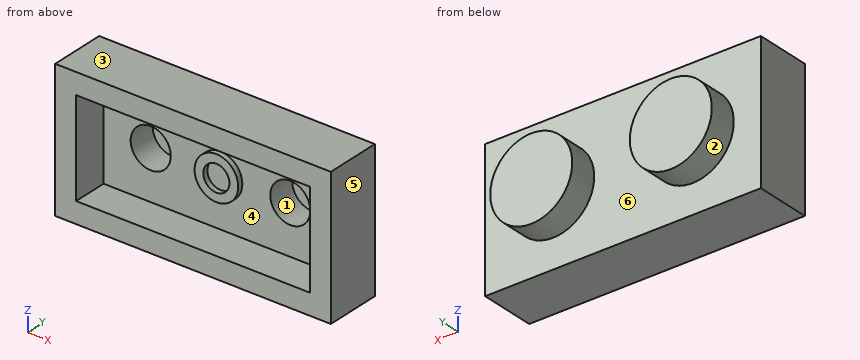
```python
from build123d import *

# Parameters (mm, degrees)
MAINBASESKETCH_W        = 15.8
MAINBASESKETCH_H        = 3.2
MAINBASEEXTRUDE_DEPTH   = 7.9
STUDSSKETCH_R           = 2.35
STUDSEXTRUDE_DEPTH      = 1.6
STUDSPATTERN_COUNT      = 2
STUDSPATTERN_PITCH      = 8
STUDSPATTERN_COUNT_DIR2 = 2
STUDSPATTERN_PITCH_DIR2 = 8
MAINBASESHELL_T         = -1.2
LCUTBLUE_DEPTH          = 19.555463972
LCUTBLUE_DEPTH_BACK     = 19.555463972
CUTADDEDTOLCUT_DEPTH    = 2
MADESLIMCUTSKETCH_W     = 7.9
MADESLIMCUTSKETCH_H     = 7.9
MADESLIMCUT_DEPTH       = 19.897228453
MADESLIMFILLEXT_REACH   = 20.897
SKETCH33_W              = 5.500952983
SKETCH33_H              = 1.199047018
SLIMHOLEEXT_START       = -0.2
SLIMHOLESKETCH_R        = 1.25
SLIMHOLESKETCH_R_2      = 0.75
SLIMHOLEEXT_DEPTH       = 0.5


with BuildPart() as part:
    # MainBaseSketch → MainBaseExtrude (new, symmetric)
    with BuildSketch(Plane.XY):
        with Locations((8.581967213, 1.6)):
            Rectangle(MAINBASESKETCH_W, MAINBASESKETCH_H)
    extrude(amount=MAINBASEEXTRUDE_DEPTH, both=True)

    # StudsSketch → StudsExtrude (add)
    with BuildSketch(Plane(origin=(0, 3.2, 0), x_dir=(1, 0, 0), z_dir=(0, 1, 0))):
        with Locations((4.581967213, 4)):
            Circle(STUDSSKETCH_R)
    studsextrude = extrude(amount=STUDSEXTRUDE_DEPTH)

    # StudsPattern: StudsExtrude 2 × 2
    with Locations(*[(j * STUDSPATTERN_PITCH_DIR2, 0, i * STUDSPATTERN_PITCH) for i in range(STUDSPATTERN_COUNT) for j in range(STUDSPATTERN_COUNT_DIR2) if (i, j) != (0, 0)]):
        add(studsextrude)

    # MainBaseShell
    mainbaseshell_openings = [part.faces().sort_by_distance(p)[0] for p in [
        (8.581967213, 0, 0),
    ]]
    offset(amount=MAINBASESHELL_T, openings=mainbaseshell_openings, kind=Kind.INTERSECTION)

    # LCUTBlueSketch → LCutBlue (cut, two sides: drawn at the far end of the back side and taken through both)
    with BuildSketch(Plane(origin=(0, 3.2, 0), x_dir=(1, 0, 0), z_dir=(0, 1, 0)).offset(-LCUTBLUE_DEPTH_BACK)):
        Polygon((8.581967213, 53.229874044), (8.581967213, 7.9), (8.581967213, 0), (16.481967213, 0), (61.811841258, 0), (125.917963912, 64.106122654), (72.688089868, 117.335996699), align=None)
    extrude(amount=LCUTBLUE_DEPTH + LCUTBLUE_DEPTH_BACK, mode=Mode.SUBTRACT)

    # CutAddedtoLSketch → CutAddedToLCut (add)
    with BuildSketch(Plane.XZ):
        Polygon((7.382920196, -6.7), (8.581967213, -6.7), (8.581967213, 0), (15.281967213, 0), (15.281967213, 1.199047018), (7.382920196, 1.199047018), (7.382920196, 0), align=None)
    extrude(amount=-CUTADDEDTOLCUT_DEPTH)

    # MadeSlimCutSketch → MadeSlimCut (cut, through all)
    with BuildSketch(Plane.XZ):
        with Locations((4.631967213, -3.95)):
            Rectangle(MADESLIMCUTSKETCH_W, MADESLIMCUTSKETCH_H)
    extrude(amount=-MADESLIMCUT_DEPTH, mode=Mode.SUBTRACT)

    # Sketch33 → MadeSlimFillExt (add, up to next)
    with BuildSketch(Plane.XZ, mode=Mode.PRIVATE) as madeslimfillext_sk1:
        with Locations((4.632443704, 0.599523509)):
            Rectangle(SKETCH33_W, SKETCH33_H)
    madeslimfillext_tool1 = extrude(madeslimfillext_sk1.sketch, amount=-MADESLIMFILLEXT_REACH, mode=Mode.PRIVATE) - part.part
    add(madeslimfillext_tool1.solids().sort_by_distance((4.632444, 0, 0.599524))[0])

    # SlimHoleSketch → SlimHoleExt (add)
    with BuildSketch(Plane.XZ.offset(-2).offset(SLIMHOLEEXT_START)):
        with Locations((8.581967213, 4)):
            Circle(SLIMHOLESKETCH_R)
        with Locations((8.581967213, 4)):
            Circle(SLIMHOLESKETCH_R_2, mode=Mode.SUBTRACT)
    extrude(amount=SLIMHOLEEXT_DEPTH)


solid = part.part
```
CAD build for the part. Positions are in the model's coordinates, mm. Face numbers are marked on the shaded views. A direction names the side the tool comes from. Coordinates: 2 decimals unless noted, no trailing zeros. Write each loop counter-clockwise with the first axis right and the second up, starting at its lowest first coordinate (ties: lowest second). Pieces come first, ordered by that corner, then holes.
(1) Cut at C-C, the plane z = 6.5. List the corners of the cut face in (x, y), and give its area (3 significant figures).
(2) Flat gauge pins, fed straight in: pin 1 (0.7 mm diameter, centred on x = 13, z = 4, fed in from -Y); pin 2 (2 mm diameter, centred on x = 8.58, z = 4, fed in from +Y); pin 3 (1 mm diameter, centred on x = 7.5, z = 2, fed in from -Y). Where does each tip first touch, or does it go through?
(3) Cut at D-D, the plane x = 14.25. List the corners of the cut face in (y, z), and give its area (3 significant figures).
(4) 3-axis set-ups, long thin cutter, end or side, ignore diameter. For the marked faces 4, 5 and 6: which of +Z, -Z, +X, -X, +Y, -Y reach the whole face in a straight line?
(5) Cut at B-B, the plane y = 2.6. List the corners of the cut face in (x, z).
(6) Drill centre lines: probe 1 along Z at (x, y) = (5.5, 1.1); probe 2 along X at (y, z) = (1.9, 4); probe 3 along X at (y, z) = (1.85, 3.5). Where is each one in solid material? Low to high.
(7) Cut at A-A, the plane y = 0.45. List the corners of the cut face in (x, z), and give its area (3 significant figures).
(8) Two-plate mould, pull along Z, no slides. Class the marked faces 1, 2 and 3: +Z half, -Z half, draft (parallel to the pull), parting line (faces both ways), or undercut.
Geometry says:
1. outline: (0.68, 0) - (1.88, 0) - (1.88, 2) - (15.28, 2) - (15.28, 0) - (16.48, 0) - (16.48, 3.2) - (0.68, 3.2) - close
1. area: 23.8 mm2
2. pin 1: stops at y = 3.6
2. pin 2: stops at y = 3.2
2. pin 3: stops at y = 2
3. outline: (0, 0) - (3.2, 0) - (3.2, 2.34) - (4.8, 2.34) - (4.8, 5.66) - (3.2, 5.66) - (3.2, 7.9) - (0, 7.9) - (0, 6.7) - (2, 6.7) - (2, 1.2) - (0, 1.2) - close
3. area: 19.6 mm2
4. face 4: -Y
4. face 5: +Z, -Z, +X, +Y, -Y
4. face 6: +Y
5. outline: (0.68, 0) - (16.48, 0) - (16.48, 7.9) - (0.68, 7.9) - close; hole circle Ø2.3 at (4.58, 4); hole circle Ø2.3 at (12.58, 4)
6. probe 1: z = 0 to 1.2, 6.7 to 7.9
6. probe 2: x = 0.68 to 1.88, 7.33 to 7.83, 9.33 to 9.83, 15.28 to 16.48
6. probe 3: x = 0.68 to 1.88, 7.44 to 8.02, 9.14 to 9.73, 15.28 to 16.48
7. outline: (0.68, 0) - (16.48, 0) - (16.48, 7.9) - (0.68, 7.9) - close; hole (1.88, 1.2) - (15.28, 1.2) - (15.28, 6.7) - (1.88, 6.7) - close
7. area: 51.1 mm2
8. face 1: undercut
8. face 2: parting line
8. face 3: +Z half
